Autodesk Inventor part; units mm, degrees
ref_plane "YZ Plane" through (0, 0, 0) normal (1, 0, 0) x (0, 1, 0)
ref_plane "XZ Plane" through (0, 0, 0) normal (0, 1, 0) x (-1, 0, 0)
ref_plane "XY Plane" through (0, 0, 0) normal (0, 0, 1) x (1, 0, 0)
sketch "Sketch1" plane through (0, 0, 0) normal (0, 0, 1) x (1, 0, 0)
  line L0 (4.1244, 7.1437) -> (8.2489, 0)
  line L1 (8.2489, 0) -> (4.1244, -7.1438)
  line L2 (4.1244, -7.1438) -> (-4.1244, -7.1437)
  line L3 (-4.1244, -7.1437) -> (-8.2489, 0)
  line L4 (-8.2489, 0) -> (-4.1244, 7.1437)
  line L5 (-4.1244, 7.1437) -> (4.1244, 7.1437)
  point P0 (0, 0)
  point P1 (0, 0)
  dimension "d0" = 14.2875
extrude "Extrusion1" add sketch "Sketch1" along normal blind 6.35
sketch "Sketch2" plane through (0, 0, 0) normal (0, 0, -1) x (-1, 0, 0)
  circle A0 centre (0, 0) radius 4.7625
  dimension "d3" = 9.525
extrude "Extrusion2" add sketch "Sketch2" along normal blind 38.1
properties part number "bolt" material "Steel, Galvanized"
Source: CAD feature listing. Evaluate the final solid. Frame: model axes, mm. A direction names the side the tool comes from. Give positions to 0.01 mm unless a question says otherwise; leave off trailing zeros. Loops run counter-clockwise (first coordinate to the right, second up) from the corner with the lowest first, then second, coordinate; pieces in that order, holes last. Notation, with made-up numbers: (51, 73.5) -> (82, 73.5) arc R29 ccw to (82, 99.5) -> close; hole circle Ø6 at (83, -0.75). An arc over 180 degrees is marked (long way). Put each result on its own line as item: value. Start each with the question number.
1) Cut plane A-A (x = 2.25). Return loops of the section in (y, z), then the cut area to 3 significant figures.
2) Contact query for flat-ended pins moving along their axis: P1, Ø1.5, axis at y = 4.5, z = -7.5, coming from the +X side; P2, Ø6, axis at x = 1.5, z = -25.5, coming from the -Y side; P3, Ø6, axis at y = -4, z = -28.5, coming from the -X side. Output: stop coordinate, or through.
3) Reachability of faces 1 (the face through (6.16, 3.62, 3.13)), 2 (the face through (4, 3, 0)) from +Z, -Z, +X, -X, +Y, -Y: full face, straight path, thin tool, end or side. Return the list, or none.
4) Material intervals for probe 1 along Z at (x, y) = (3, 4.25); probe 2 along Y at (x, z) = (-7, 1); probe 3 along X at (y, z) = (0.5, -13), sorted ascending.
5) Cut plane C-C (y = 3.5). Return loops of the section in (x, z), then the cut area to 3 significant figures.
6) Cut plane B-B (z = -17.5). Return loops of the section in (x, y) (1 decimal), then the cut area to 3 significant figures.
7) Cut plane D-D (x = -5.5). Return loops of the section in (y, z), then the cut area to 3 significant figures.
Results are:
1. outline: (-7.14, 0) -> (-4.2, 0) -> (-4.2, -38.1) -> (4.2, -38.1) -> (4.2, 0) -> (7.14, 0) -> (7.14, 6.35) -> (-7.14, 6.35) -> close
1. area: 411 mm2
2. P1: stops at x = 2.94
2. P2: stops at y = -4.76
2. P3: stops at x = -4.66
3. face 1: +Z, -Z, +X, +Y
3. face 2: -Z
4. probe 1: z = 0 to 6.35
4. probe 2: y = -2.16 to 2.16
4. probe 3: x = -4.74 to 4.74
5. outline: (-6.23, 0) -> (-3.23, 0) -> (-3.23, -38.1) -> (3.23, -38.1) -> (3.23, 0) -> (6.23, 0) -> (6.23, 6.35) -> (-6.23, 6.35) -> close
5. area: 325 mm2
6. outline: circle Ø9.5 at (0, 0)
6. area: 71.3 mm2
7. outline: (-4.76, 0) -> (4.76, 0) -> (4.76, 6.35) -> (-4.76, 6.35) -> close
7. area: 60.5 mm2
